```python
from build123d import *

# Parameters (mm, degrees)
SKETCH1_R               = 6.25
BOSS_EXTRUDE1_DEPTH     = 25.1
SKETCH3_R               = 47.5
CUT_EXTRUDE2_DEPTH      = 14
CUT_EXTRUDE5_DEPTH      = 332.443826311
CUT_EXTRUDE5_DEPTH_BACK = 332.443826311
SKETCH2_R               = 2.494998654
SKETCH2_R_2             = 2.5
SKETCH2_R_3             = 2.444443829
SKETCH6_R               = 3
CUT_EXTRUDE6_DEPTH      = 6
CUT_EXTRUDE7_DEPTH      = 331.788452035
CUT_EXTRUDE7_DEPTH_BACK = 331.788452035
FILLET1_R               = 200
FILLET2_R               = 3


with BuildPart() as part:
    # Sketch1 → Boss-Extrude1 (new body)
    with BuildSketch(Plane.XY):
        with BuildLine():
            Line((54.543560573, 25), (300, 25))
            ThreePointArc((300, 25), (325, 0), (300, -25))
            Line((300, -25), (54.543560573, -25))
            ThreePointArc((54.543560573, -25), (-60, 0), (54.543560573, 25))
        make_face()
        with Locations((300, 0)):
            Circle(SKETCH1_R, mode=Mode.SUBTRACT)
    extrude(amount=BOSS_EXTRUDE1_DEPTH)

    # Sketch3 → Cut-Extrude2 (cut)
    with BuildSketch(Plane.XY.offset(25.1)):
        Circle(SKETCH3_R)
    extrude(amount=-CUT_EXTRUDE2_DEPTH, mode=Mode.SUBTRACT)

    # Sketch2 → Cut-Extrude5 (cut, two sides: drawn at the far end of the back side and taken through both)
    with BuildSketch(Plane.XY.offset(25.1).offset(-CUT_EXTRUDE5_DEPTH_BACK)):
        with Locations((-16.664697145, -50.733104448)):
            Circle(SKETCH2_R)
        with Locations((-50.733105114, 16.664696544)):
            Circle(SKETCH2_R_2)
        with Locations((16.664695878, 50.733104512)):
            Circle(SKETCH2_R_3)
        with Locations((50.733103846, -16.66469648)):
            Circle(SKETCH2_R_2)
    extrude(amount=CUT_EXTRUDE5_DEPTH + CUT_EXTRUDE5_DEPTH_BACK, mode=Mode.SUBTRACT)

    # Sketch6 → Cut-Extrude6 (cut)
    with BuildSketch(Plane(origin=(0, 0, 0), x_dir=(-1, 0, 0), z_dir=(0, 0, -1))):
        with Locations((11.973502988, 47.212610548)):
            Circle(SKETCH6_R)
        with Locations((27.381285989, 40.029281029)):
            Circle(SKETCH6_R)
        with Locations((-19.717656658, -20.762902692)):
            Circle(SKETCH6_R)
        with Locations((-4.309873657, -27.946232212)):
            Circle(SKETCH6_R)
    extrude(amount=-CUT_EXTRUDE6_DEPTH, mode=Mode.SUBTRACT)

    # Sketch7 → Cut-Extrude7 (cut, two sides: drawn at the far end of the back side and taken through both)
    with BuildSketch(Plane.XY.offset(11.1).offset(-CUT_EXTRUDE7_DEPTH_BACK)):
        Polygon((-32.400942803, 32.871850778), (-3.10901045, -26.912408633), (24.254242539, -13.505492441), (-3.650778768, 46.958298756), align=None)
    extrude(amount=CUT_EXTRUDE7_DEPTH + CUT_EXTRUDE7_DEPTH_BACK, mode=Mode.SUBTRACT)

    # Fillet1
    fillet1_edges = [part.edges().sort_by_distance(p)[0] for p in [
        (54.543560573, 25, 12.55),
        (54.543560573, -25, 12.55),
    ]]
    fillet(fillet1_edges, radius=FILLET1_R)

    # Fillet2
    fillet2_edges = [part.edges().sort_by_distance(p)[0] for p in [
        (325, 0, 25.1),
        (215.144071104, 25, 25.1),
        (215.144071104, 25, 0),
        (325, 0, 0),
        (215.144071104, -25, 0),
        (215.144071104, -25, 25.1),
        (-60, 0, 0),
        (-60, 0, 25.1),
        (78.400690042, -31.848007239, 0),
        (78.400690042, -31.848007239, 25.1),
        (78.400690042, 31.848007239, 0),
        (78.400690042, 31.848007239, 25.1),
    ]]
    fillet(fillet2_edges, radius=FILLET2_R)


solid = part.part
```
CAD build for the part. Positions are in the model's coordinates, mm. A direction names the side the tool comes from. Give positions to 0.01 mm unless a question says otherwise; leave off trailing zeros. Order: outer loops, then holes, each group sorted by start corner. A loop starts at its lowest first (then second) coordinate and runs counter-clockwise, first axis right, second up.
(1) Tool access for faces 5 (the flat face through (214, 25, 12)), 6 (the flat face through (-17.825, 40.014, 5.472)), 7 (the flat face through (216, -25, 12)): list every direction of +Z, -Z, +X, -X, +Y, -Y with a clear straight run to the whole face (end or side of a thin tool).
(2) Drill centre lines: L1, parallel to Y at x = 1, z = 21; L2, parallel to X at y = -3, z = 18.25; L3, parallel to Y at x = 144, z = 12.5. Where is each one in solid material? Low to high.
(3) Mould opens along Y. For faces 1 (the flat face through (147, -4, 25.1)), 2 (the flat face through (20, 1, 11.1)), 3 (the flat face through (10.381, -20.303, 5.472)), 4 (the cylindrical face through (79.11, 31.66, 12.68)) say: released by +Y, released by -Y, zero draft, split by the parting line, or undercut.
(4) Flat gauge pins, fed straight in: pin 1 (1 mm diameter, centred on x = 208.5, z = 13.5, fed in from -Y); pin 2 (2 mm diameter, centred on x = 254, z = 7.5, fed in from +Y); pin 3 (1.8 mm diameter, centred on x = 3, y = -27, fed in from -Z). Where does each tip first touch, or does it go through?
(5) Saw through at A-A, the plane x = 165. Give the cut face in (y, z).
(6) Saw through at B-B, the plane y = 0. Give the cut face in (x, z).
Results found:
1. face 5: +Z, -Z, +X, +Y
1. face 6: +Z, -Z
1. face 7: +Z, -Z, +X, -Y
2. L1: y = -59.99 to -47.49, 47.49 to 59.99
2. L2: x = -59.92 to -47.41, 47.41 to 294.52, 305.48 to 324.82
2. L3: y = -25 to 25
3. face 1: zero draft
3. face 2: undercut
3. face 3: undercut
3. face 4: released by +Y
4. pin 1: stops at y = -25
4. pin 2: stops at y = 25
4. pin 3: stops at z = 6
5. outline: (-25, 3) arc R3 ccw to (-22, 0) - (22, 0) arc R3 ccw to (25, 3) - (25, 22.1) arc R3 ccw to (22, 25.1) - (-22, 25.1) arc R3 ccw to (-25, 22.1) - close
6. outline: (-60, 3) arc R3 ccw to (-57, 0) - (-16.3, 0) - (-16.3, 11.1) - (-47.5, 11.1) - (-47.5, 25.1) - (-57, 25.1) arc R3 ccw to (-60, 22.1) - close; (18.02, 0) - (293.75, 0) - (293.75, 25.1) - (47.5, 25.1) - (47.5, 11.1) - (18.02, 11.1) - close; (306.25, 0) - (322, 0) arc R3 ccw to (325, 3) - (325, 22.1) arc R3 ccw to (322, 25.1) - (306.25, 25.1) - close
